Can you work these out from the model? Positions are in its coordinate system, mm. A direction names the side the tool comes from. Round coordinates to 2 decimals unless told otherwise and drop trailing zeros. Order: outer loops, then holes, each group sorted by start corner. A loop starts at its lowest first (then second) coordinate and runs counter-clockwise, first axis right, second up.
Q1. If we section it at A-A (z = 8.25): Please give me the cut outline in (x, y) (3 decimals).
Q2. For faces 1 (the face through (-22.213, 0.558, 6.261)), 2 (the face through (14, 0, 2.54)), which set-ups out of +Z, -Z, +X, -X, +Y, -Y let a thin tool reach every point of the face, with its end or its side?
Q3. Will these pins go through, and if not, where does the flat tip stop? P1, Ø2, axis at x = -13, z = 6, coming from the -Y side; P2, Ø1.5, axis at x = -0.5, y = 13.5, coming from the +Z side; P3, Ø7, axis at y = 7, z = 9.5, coming from the -X side.
Q4. If we section it at B-B (y = 0): Please give me the cut outline in (x, z) (3 decimals).
Q5. We'd pull the mould along X, two halves only. Please class faces 3 (the face through (28.575, 0, 6)), 4 (the face through (13, -8, 12.7)), 5 (the face through (-21.6, -9.3, 8.2)): pulls with the +X half, pulls with the -X half, needs draft (parallel to the pull), parting line crosses it, or undercut.
Q6. If we section it at C-C (y = -11): Count the separate pieces of the cut face and the enclosed holes in it, plus the area to 3 significant figures.
Q7. If I drill on line 1 (Y direction, x = -11.5, z = 10); line 2 (Y direction, x = 26, z = 11.5); line 3 (X direction, y = 9, z = 5.5) (3 decimals), over which ranges is the centre line in solid material (lowest first)?
from build123d import *

# Parameters (mm, degrees)
F0_R         = 3.175
F0_R_2       = 12.7
F1_DEPTH     = 12.7
F2_T         = -2.54
F3_T1_DEPTH  = 33.02
F3_T6_DEPTH  = 24.3152905029
F3_S7_R      = 5.715
F3_T8_DEPTH  = 14
F3_T12_ANGLE = 253.7190819507
F3_T17_ANGLE = 73.6440624835
F3_T22_DEPTH = 9.0752905029
F3_S23_R     = 5.715
F3_T24_DEPTH = 6
F3_T28_DEPTH = 9.0752905029
F3_S29_R     = 5.715
F3_T30_DEPTH = 6
F3_T34_ANGLE = 73.6440624835
F3_T39_ANGLE = 253.7190819507
F3_T44_DEPTH = 24.3152905029
F3_S45_R     = 5.715
F3_T46_DEPTH = 14
F3_T48_ANGLE = 180


# Not quite as in the source:
# - a fillet or chamfer that OpenCascade refuses, or shapes differently, is made with other operations: its cross-section is extruded or revolved along the edge and cut away or added


with BuildPart() as f1:
    # F0 (on Top) → F1 (new body)
    with BuildSketch(Plane.XY):
        with BuildLine():
            Line((28.575, -19.05), (28.575, 19.05))
            Line((28.575, 19.05), (-9.525, 19.05))
            ThreePointArc((-9.525, 19.05), (-28.575, 0), (-9.525, -19.05))
            Line((-9.525, -19.05), (28.575, -19.05))
        make_face()
        with Locations((15.875, -12.7)):
            Circle(F0_R, mode=Mode.SUBTRACT)
        with Locations((-9.525, 0)):
            Circle(F0_R_2, mode=Mode.SUBTRACT)
        with Locations((15.875, 12.7)):
            Circle(F0_R, mode=Mode.SUBTRACT)
    extrude(amount=F1_DEPTH)

    # F2
    f2_openings = [f1.faces().sort_by_distance(p)[0] for p in [
        (5.241716, 0, 12.7),
    ]]
    offset(amount=F2_T, openings=f2_openings)

    # F3: fillet of radius 1.27 on 11 edges, made by hand

    # F3_s2 → F3_t1 (join)
    with BuildSketch(Plane.XZ.offset(-16.51)):
        with BuildLine():
            ThreePointArc((26.035, 3.81), (25.6630256121, 2.9119743879), (24.765, 2.54))
            Line((24.765, 2.54), (26.035, 2.54))
            Line((26.035, 2.54), (26.035, 3.81))
        make_face()
    extrude(amount=F3_T1_DEPTH)


with BuildPart() as f3_tool4:
    # F3_s5 → F3_t6 (new body)
    with BuildSketch(Plane.YZ.offset(-9.525)):
        with BuildLine():
            ThreePointArc((-16.51, 3.81), (-16.1380256121, 2.9119743879), (-15.24, 2.54))
            Line((-15.24, 2.54), (-16.51, 2.54))
            Line((-16.51, 2.54), (-16.51, 3.81))
        make_face()
    extrude(amount=F3_T6_DEPTH)

    # F3_s7 → F3_t8 (cut, symmetric)
    with BuildSketch(Plane.XY.offset(3.2)):
        with Locations((15.875, -12.7)):
            Circle(F3_S7_R)
    extrude(amount=F3_T8_DEPTH, both=True, mode=Mode.SUBTRACT)


with BuildPart() as f1_1:
    add(f1.part)

    # F3_t3: union F3_tool4
    add(f3_tool4.part)


with BuildPart() as f3_tool10:
    # F3_s11 → F3_t12 (revolve)
    with BuildSketch(Plane(origin=(18.0449433807, -5.2701877221, 0), x_dir=(0, 0, 1), z_dir=(0.9598987128, -0.2803470371, 0))):
        with BuildLine():
            ThreePointArc((3.81, 13.4552044392), (2.9119743879, 13.8271788271), (2.54, 14.7252044392))
            Line((2.54, 14.7252044392), (2.54, 13.4552044392))
            Line((2.54, 13.4552044392), (3.81, 13.4552044392))
        make_face()
    revolve(axis=Axis((15.875, -12.7, 2.54), (0, 0, -1)), revolution_arc=F3_T12_ANGLE)

    split(bisect_by=Plane.XZ.offset(16.51), keep=Keep.BOTTOM)


with BuildPart() as f1_2:
    add(f1_1.part)

    # F3_t9: union F3_tool10
    add(f3_tool10.part)


with BuildPart() as f3_tool15:
    # F3_s16 → F3_t17 (revolve)
    with BuildSketch(Plane.XZ.offset(12.7)):
        with BuildLine():
            ThreePointArc((21.59, 3.81), (21.9619743879, 2.9119743879), (22.86, 2.54))
            Line((22.86, 2.54), (21.59, 2.54))
            Line((21.59, 2.54), (21.59, 3.81))
        make_face()
    revolve(axis=Axis((15.875, -12.7, 2.54), (0, 0, -1)), revolution_arc=F3_T17_ANGLE)

    split(bisect_by=Plane.XZ.offset(16.51), keep=Keep.BOTTOM)


with BuildPart() as f1_3:
    add(f1_2.part)

    # F3_t14: union F3_tool15
    add(f3_tool15.part)


with BuildPart() as f3_tool20:
    # F3_s21 → F3_t22 (new body)
    with BuildSketch(Plane.YZ.offset(16.9597094971)):
        with BuildLine():
            ThreePointArc((-16.51, 3.81), (-16.1380256121, 2.9119743879), (-15.24, 2.54))
            Line((-15.24, 2.54), (-16.51, 2.54))
            Line((-16.51, 2.54), (-16.51, 3.81))
        make_face()
    extrude(amount=F3_T22_DEPTH)

    # F3_s23 → F3_t24 (cut, symmetric)
    with BuildSketch(Plane.XY.offset(3.2)):
        with Locations((15.875, -12.7)):
            Circle(F3_S23_R)
    extrude(amount=F3_T24_DEPTH, both=True, mode=Mode.SUBTRACT)


with BuildPart() as f1_4:
    add(f1_3.part)

    # F3_t19: union F3_tool20
    add(f3_tool20.part)


with BuildPart() as f3_tool26:
    # F3_s27 → F3_t28 (new body)
    with BuildSketch(Plane.YZ.offset(26.035)):
        with BuildLine():
            ThreePointArc((16.51, 3.81), (16.1380256121, 2.9119743879), (15.24, 2.54))
            Line((15.24, 2.54), (16.51, 2.54))
            Line((16.51, 2.54), (16.51, 3.81))
        make_face()
    extrude(amount=-F3_T28_DEPTH)

    # F3_s29 → F3_t30 (cut, symmetric)
    with BuildSketch(Plane.XY.offset(3.2)):
        with Locations((15.875, 12.7)):
            Circle(F3_S29_R)
    extrude(amount=F3_T30_DEPTH, both=True, mode=Mode.SUBTRACT)


with BuildPart() as f1_5:
    add(f1_4.part)

    # F3_t25: union F3_tool26
    add(f3_tool26.part)


with BuildPart() as f3_tool32:
    # F3_s33 → F3_t34 (revolve)
    with BuildSketch(Plane(origin=(11.1844694654, -3.2824241778, 0), x_dir=(0, 0, 1), z_dir=(-0.9595308214, 0.281603627, 0))):
        with BuildLine():
            ThreePointArc((3.81, 22.3714990108), (2.9119743879, 22.7434733987), (2.54, 23.6414990108))
            Line((2.54, 23.6414990108), (2.54, 22.3714990108))
            Line((2.54, 22.3714990108), (3.81, 22.3714990108))
        make_face()
    revolve(axis=Axis((15.875, 12.7, 2.54), (0, 0, -1)), revolution_arc=F3_T34_ANGLE)

    split(bisect_by=Plane.XZ.offset(-16.51), keep=Keep.TOP)


with BuildPart() as f1_6:
    add(f1_5.part)

    # F3_t31: union F3_tool32
    add(f3_tool32.part)


with BuildPart() as f3_tool37:
    # F3_s38 → F3_t39 (revolve)
    with BuildSketch(Plane.XZ.offset(-12.7)):
        with BuildLine():
            ThreePointArc((21.59, 3.81), (21.9619743879, 2.9119743879), (22.86, 2.54))
            Line((22.86, 2.54), (21.59, 2.54))
            Line((21.59, 2.54), (21.59, 3.81))
        make_face()
    revolve(axis=Axis((15.875, 12.7, 2.54), (0, 0, -1)), revolution_arc=F3_T39_ANGLE)

    split(bisect_by=Plane.XZ.offset(-16.51), keep=Keep.TOP)


with BuildPart() as f1_7:
    add(f1_6.part)

    # F3_t36: union F3_tool37
    add(f3_tool37.part)


with BuildPart() as f3_tool42:
    # F3_s43 → F3_t44 (new body)
    with BuildSketch(Plane.YZ.offset(14.7902905029)):
        with BuildLine():
            ThreePointArc((16.51, 3.81), (16.1380256121, 2.9119743879), (15.24, 2.54))
            Line((15.24, 2.54), (16.51, 2.54))
            Line((16.51, 2.54), (16.51, 3.81))
        make_face()
    extrude(amount=-F3_T44_DEPTH)

    # F3_s45 → F3_t46 (cut, symmetric)
    with BuildSketch(Plane.XY.offset(3.2)):
        with Locations((15.875, 12.7)):
            Circle(F3_S45_R)
    extrude(amount=F3_T46_DEPTH, both=True, mode=Mode.SUBTRACT)


with BuildPart() as f1_8:
    add(f1_7.part)

    # F3_t41: union F3_tool42
    add(f3_tool42.part)

    # F3_s47 → F3_t48 (revolve)
    with BuildSketch(Plane.YZ.offset(-9.525)):
        with BuildLine():
            ThreePointArc((-16.51, 3.81), (-16.1380256121, 2.9119743879), (-15.24, 2.54))
            Line((-15.24, 2.54), (-16.51, 2.54))
            Line((-16.51, 2.54), (-16.51, 3.81))
        make_face()
    revolve(axis=Axis((-9.525, 0, 2.54), (0, 0, -1)), revolution_arc=F3_T48_ANGLE)

    # F3_s49 → F3_t50 (revolve)
    with BuildSketch(Plane.XZ):
        with BuildLine():
            ThreePointArc((6.985, 2.54), (6.0869743879, 2.9119743879), (5.715, 3.81))
            Line((5.715, 3.81), (5.715, 2.54))
            Line((5.715, 2.54), (6.985, 2.54))
        make_face()
    revolve(axis=Axis((-9.525, 0, 2.54), (0, 0, -1)))


solid = f1_8.part
Solution:
1. outline: circle Ø30.48 at (-9.525, 0); (-9.525, -19.05) - (28.575, -19.05) - (28.575, 19.05) - (-9.525, 19.05) arc R19.05 ccw to start; hole circle Ø25.4 at (-9.525, 0); hole (-9.525, -16.51) - (11.615, -16.51) arc R5.715 cw (long way) to (20.135, -16.51) - (26.035, -16.51) - (26.035, 16.51) - (20.135, 16.51) arc R5.715 cw (long way) to (11.615, 16.51) - (-9.525, 16.51) arc R16.51 ccw to start; hole circle Ø6.35 at (15.875, -12.7); hole circle Ø6.35 at (15.875, 12.7)
2. face 1: +Z, -Z
2. face 2: +Z
3. P1: stops at y = -18.89
3. P2: stops at z = 3.05
3. P3: stops at x = -28.25
4. outline: (-28.575, 0) - (-22.225, 0) - (-22.225, 12.7) - (-24.765, 12.7) - (-24.765, 3.81) arc R1.27 cw to (-25.4, 2.71) arc R1.27 cw to (-26.035, 3.81) - (-26.035, 12.7) - (-28.575, 12.7) - close; (3.175, 0) - (28.575, 0) - (28.575, 12.7) - (26.035, 12.7) - (26.035, 3.81) arc R1.27 cw to (24.765, 2.54) - (6.985, 2.54) arc R1.27 cw to (5.715, 3.81) - (5.715, 12.7) - (3.175, 12.7) - close
5. face 3: pulls with the +X half
5. face 4: needs draft
5. face 5: undercut
6. separate pieces: 3
6. enclosed holes: 0
6. area: 293 mm2
7. line 1: y = -18.95 to -16.39, -15.11 to -12.55, 12.55 to 15.11, 16.39 to 18.95
7. line 2: y = -19.05 to -16.51, 16.51 to 19.05
7. line 3: x = -26.315 to -23.366, -21.824 to -18.485, -0.565 to 2.774, 11.519 to 20.231, 26.035 to 28.575
